Autodesk Inventor part; units mm, degrees
ref_plane "YZ Plane" through (0, 0, 0) normal (1, 0, 0) x (0, 1, 0)
ref_plane "XZ Plane" through (0, 0, 0) normal (0, 1, 0) x (-1, 0, 0)
ref_plane "XY Plane" through (0, 0, 0) normal (0, 0, 1) x (1, 0, 0)
sketch "Sketch6" plane through (0, 0, 0) normal (0, 0, 1) x (1, 0, 0)
  circle A0 centre (0, 0) radius 9
  circle A1 centre (0, 0) radius 14
  dimension "d20" = 18
  dimension "d21" = 28
extrude "Extrusion4" add sketch "Sketch6" along normal blind 35
ref_plane "Work Plane2" through (0, 0, 17.5) normal (0, 0, 1) x (1, 0, 0)
sketch "Sketch8" plane through (0, 0, 17.5) normal (0, 0, 1) x (1, 0, 0)
  line L0 (0, 0) -> (0, 26)
  line L1 (0, 26) -> (-9.5, 26)
  line L2 (-9.5, 26) -> (-9.5, 21.5)
  line L3 (-9.5, 21.5) -> (0, 21.5)
  line L4 (0, 21.5) -> (0, 26)
  line L5 (0, 21.5) -> (-9.5, 21.5)
  line L6 (-9.5, 21.5) -> (-9.5, 18.5)
  line L7 (-9.5, 18.5) -> (0, 18.5)
  line L8 (0, 18.5) -> (0, 21.5)
  line L9 (9.5, 21.5) -> (0, 21.5)
  line L10 (9.5, 21.5) -> (9.5, 18.5)
  line L11 (9.5, 18.5) -> (0, 18.5)
  dimension "d28" = 26
  dimension "d29" = 9.5
  dimension "d30" = 4.5
  dimension "d32" = 3
revolve "Revolution1" add sketch "Sketch8" angle 360 about axis through (0, 26, 17.5) along (-1, 0, 0) contours L7 L6 L3 L0 | L0 L9 L10 L11
sketch "Sketch10" plane through (0, 0, 17.5) normal (0, 0, 1) x (1, 0, 0)
  circle A0 centre (0, 0) radius 14
  line L0 (-14, 0) -> (-9.5, 19)
  line L1 (-9.5, 19) -> (0, 19)
  line L2 (-9.5, 33.5) -> (-9.5, 18.5)
  line L3 (0, 19) -> (0, 0)
  line L4 (14, 0) -> (9.5, 19)
  line L5 (9.5, 19) -> (0, 19)
  point P0 (-12.5128, 6.2793)
  point P1 (12.5128, 6.2793)
  dimension "d35" = 19
  dimension "d36" = 9.5
extrude "Extrusion6" add sketch "Sketch10" along normal blind 2.5 contours L0 L1 L3 A0 | A0 L3 L5 L4
mirror "Mirror2" about plane through (0, 0, 17.5) normal (0, 0, 1) of "Extrusion6"
ref_plane "Work Plane3" through (0, 59.1111, 15) normal (-1, 0, 0) x (0, 0, 1)
sketch "Sketch11" plane through (0, 59.1111, 15) normal (-1, 0, 0) x (0, 0, 1)
  arc A0 (5, -40.1822) -> (0, -40.1822) centre (2.5, -33.1111) ccw
  line L0 (-5, -33.1111) -> (-15, -45.1111)
  line L1 (-15, -45.1111) -> (20, -45.1111)
  circle A1 centre (2.5, -33.1111) radius 7.5
  line L2 (2.5, -33.1111) -> (2.5, -59.6944)
  line L3 (10, -33.1111) -> (20, -45.1111)
  point P0 (-15, -59.1111)
extrude "Extrusion7" add sketch "Sketch11" along normal blind 2.5 contours A0 L3 L1 L2 A1 | L2 L1 L0 A0 A1
mirror "Mirror3" about plane through (0, 59.1111, 15) normal (-1, 0, 0) of "Extrusion7"
Read the model definition and answer for the solid it produces. Units are mm, in the model's axes. A direction names the side the tool comes from. Give positions to 0.01 mm unless a question says otherwise; leave off trailing zeros. Write each loop counter-clockwise with the first axis right and the second up, starting at its lowest first coordinate (ties: lowest second). Pieces come first, ordered by that corner, then holes. Notation, with made-up numbers: (23, 38.25) -> (28, 38.25) arc R20 ccw to (28, 76.25) -> close; hole circle Ø7 at (55.5, 35.25). An arc over 180 degrees is marked (long way). Answer in a Markdown table with one row per item.
1) Determine the mould class of faces 4 (the flat face through (-10.985, 12.729, 17.535)), 5 (the cylindrical face through (-1.172, -8.923, 17.255)), 6 (the flat face through (-7, 15, 15)) for opening direction X: released by +X, released by -X, zero draft, split by the parting line, or undercut.
Results list:
| item | result |
|---|---|
| face 4 | released by -X |
| face 5 | undercut |
| face 6 | zero draft |
2) Section B-B on x = 5.75 is taken. Give the vertices of the cut face in (y, z).
Results list:
| item | result |
|---|---|
| outline | (-12.76, 0) -> (-6.92, 0) -> (-6.92, 35) -> (-12.76, 35) -> close; (6.92, 0) -> (12.76, 0) -> (12.76, 15) -> (18.93, 15) arc R7.5 ccw (long way) to (18.93, 20) -> (12.76, 20) -> (12.76, 35) -> (6.92, 35) -> close; hole circle Ø9 at (26, 17.5) |
3) Each of these flat-tipped pins is pushed along its axis until it touches: pin 1 Ø5 at (y, z) = (4.5, 6.5) entering from -X; pin 2 Ø6 at (y, z) = (18.5, 30.5) entering from -X; pin 3 Ø7.5 at (y, z) = (26.5, 14.5) entering from +X; pin 4 Ø7 at (y, z) = (26, 17.5) entering from +X. Where does it stop, or does it pass through?
Results list:
| item | result |
|---|---|
| pin 1 | x = -13.86 |
| pin 2 | x = -2.5 |
| pin 3 | x = 9.5 |
| pin 4 | through |
4) A tool of negligible diameter and unlimited length cuts with its end or side. For faces 1 (the flat face through (-9.5, 21, 18)), 2 (the cylindrical face through (0.133, 33.494, 17.206)), 3 (the flat face through (2.5, 17, 9)), from which of +Z, -Z, +X, -X, +Y, -Y can it reach the whole face along a straight path? Write none if from no direction.
Results list:
| item | result |
|---|---|
| face 1 | +Z, -Z, -X, +Y |
| face 2 | none |
| face 3 | -Z, +X |
5) Straight lines are drawn through the part: line 1 (Z direction, x = 2.5, y = 26); line 2 (Z direction, x = -7.5, y = 15.5); line 3 (X direction, y = -6.5, z = 30). For each, find the intervals that lie inside material, in ascending order. Write a range as [from, to].
Results list:
| item | result |
|---|---|
| line 1 | [10, 13], [22, 25] |
| line 2 | [15, 20] |
| line 3 | [-12.4, -6.22], [6.22, 12.4] |
6) Section C-C on y = -5.5 is taken. Give the vertices of the cut face in (x, z), plus the area to 3 significant figures.
Results list:
| item | result |
|---|---|
| outline | (-12.87, 0) -> (-7.12, 0) -> (-7.12, 35) -> (-12.87, 35) -> close; (7.12, 0) -> (12.87, 0) -> (12.87, 35) -> (7.12, 35) -> close |
| area | 403 mm^2 |
